Source: three-view drawing plus pictorial views. Frame: mm from the lowest corner of the part. Round coordinates to 2 decimals unless told otherwise and drop trailing zeros. Loops run counter-clockwise (first coordinate to the right, second up) from the corner with the lowest first, then second, coordinate; pieces in that order, holes last. Notation, with made-up numbers: M 4,20.5 L 9,20.5 A16 cw 9,43.5 Z; hole C -33,11.5 d5. An arc over 180 degrees is marked long. Return JSON: item names as keys, results as strings. Group by question number.
1) Contact query for flat-ended pins moving along their axis: P1, Ø1, axis at x = 15, z = 1.5, coming from the +Y side; P2, Ø2, axis at x = 16, z = 7.5, coming from the +Y side; P3, Ø4, axis at y = 5.5, z = 4.5, coming from the -X side. Output: stop coordinate, or through.
2) Section A-A (z = 10). Output: boundary loops of the cut face in (x, y).
3) Material intervals for line 1 (Y direction, x = 25, z = 9); line 2 (Y direction, x = 31.5, z = 5.75); line 3 (X direction, y = 7.5, z = 4.5), sorted ascending. Write a range as from..to.
4) Section B-B (x = 25). Output: boundary loops of the cut face in (y, z), plus the area to 3 significant figures.
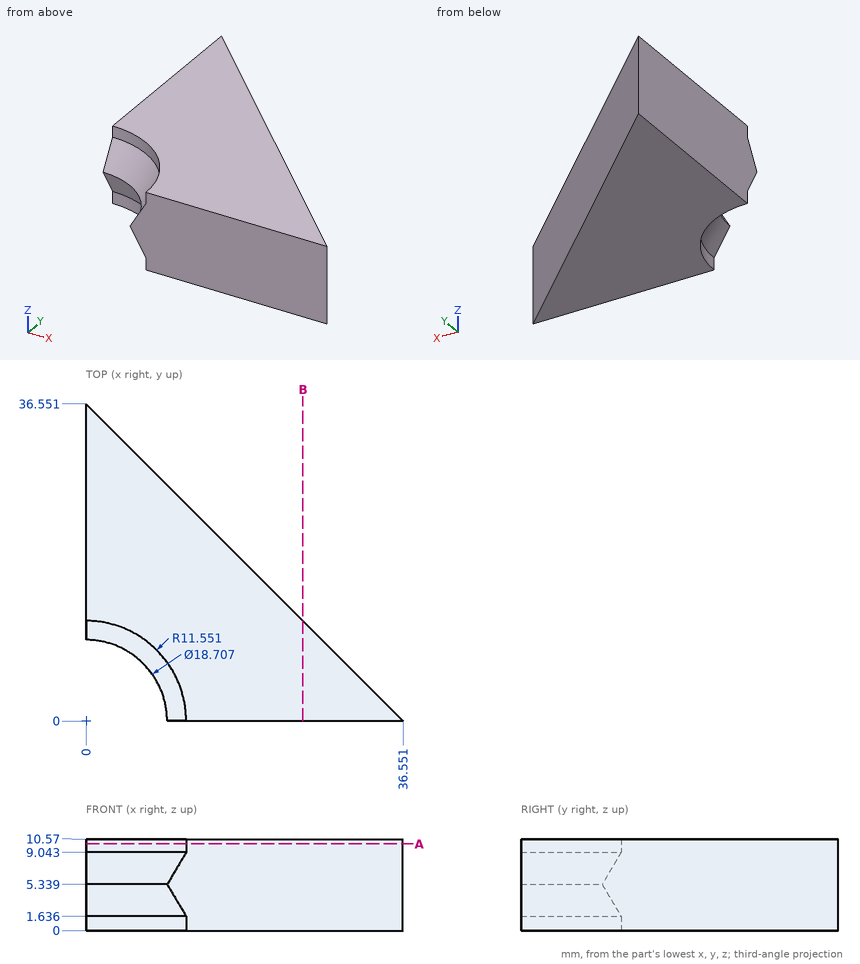
Returned:
{
 "1": {"P1": "stops at y = 22.05", "P2": "stops at y = 21.55", "P3": "stops at x = 5.83"},
 "2": {"outline": "M 0,11.55 A11.55 cw 11.55,0 L 36.55,0 L 0,36.55 Z"},
 "3": {"line 1": "y = 0..11.55", "line 2": "y = 0..5.05", "line 3": "x = 6.39..29.05"},
 "4": {"outline": "M 0,0 L 11.55,0 L 11.55,10.57 L 0,10.57 Z", "area": "122 mm^2"}
}
